```python
from build123d import *

# Parameters (mm, degrees)
SZKIC1_W                        = 203
SZKIC1_H                        = 545
DODANIE_WYCI_GNI_CIE1_DEPTH     = 1
WYTNIJ_WYCI_GNI_CIE1_DEPTH      = 437.073905415
WYTNIJ_WYCI_GNI_CIE1_DEPTH_BACK = 437.073905415
SZKIC2_W                        = 21
SZKIC2_H                        = 21
SZKIC3_W                        = 21
SZKIC3_H                        = 21
WYTNIJ_WYCI_GNI_CIE2_DEPTH      = 437.073905415
SZKIC4_W                        = 22
SZKIC4_H                        = 46.721864408
WYTNIJ_WYCI_GNI_CIE3_DEPTH      = 437.073905415
SZKIC5_W                        = 161
SZKIC5_H                        = 1
DODANIE_WYCI_GNI_CIE2_DEPTH     = 1.5
SZKIC6_R                        = 2.1
WYTNIJ_WYCI_GNI_CIE4_DEPTH      = 437.073905415
SZKIC7_R                        = 2.45
WYTNIJ_WYCI_GNI_CIE5_DEPTH      = 437.073905415
SZKIC8_W                        = 1
SZKIC8_H                        = 218.015474914
DODANIE_WYCI_GNI_CIE3_DEPTH     = 1.5
SZKIC9_W                        = 1
SZKIC9_H                        = 237.530488001
DODANIE_WYCI_GNI_CIE4_DEPTH     = 1.5
SZKIC10_R                       = 2
SZKIC10_R_2                     = 1.651116854
SZKIC10_R_3                     = 1.6
SZKIC10_R_4                     = 2.1
SZKIC10_R_5                     = 1.9
WYTNIJ_WYCI_GNI_CIE6_DEPTH      = 437.476994539
SZKIC11_R                       = 1.6
WYTNIJ_WYCI_GNI_CIE7_DEPTH      = 437.476994539
SZKIC12_R                       = 1.6
WYTNIJ_WYCI_GNI_CIE8_DEPTH      = 437.476994539


with BuildPart() as part:
    # Szkic1 → Dodanie-wyciągnięcie1 (new body)
    with BuildSketch(Plane.XY):
        with Locations((-14.988592715, -147.725961538)):
            Rectangle(SZKIC1_W, SZKIC1_H)
    extrude(amount=DODANIE_WYCI_GNI_CIE1_DEPTH)

    # Szkic2 → Wytnij-wyciągnięcie1 (cut, two sides: drawn at the far end of the back side and taken through both)
    with BuildSketch(Plane.XY.offset(1).offset(-WYTNIJ_WYCI_GNI_CIE1_DEPTH_BACK)):
        with Locations((-105.988592715, 114.274038462)):
            Rectangle(SZKIC2_W, SZKIC2_H)
        with Locations((76.011407285, 114.274038462)):
            Rectangle(SZKIC2_W, SZKIC2_H)
    extrude(amount=WYTNIJ_WYCI_GNI_CIE1_DEPTH + WYTNIJ_WYCI_GNI_CIE1_DEPTH_BACK, mode=Mode.SUBTRACT)

    # Szkic3 → Wytnij-wyciągnięcie2 (cut, through all)
    with BuildSketch(Plane.XY.offset(1)):
        with Locations((76.011407285, -409.725961538)):
            Rectangle(SZKIC3_W, SZKIC3_H)
        with Locations((-105.988592715, -409.725961538)):
            Rectangle(SZKIC3_W, SZKIC3_H)
    extrude(amount=-WYTNIJ_WYCI_GNI_CIE2_DEPTH, mode=Mode.SUBTRACT)

    # Szkic4 → Wytnij-wyciągnięcie3 (cut, through all)
    with BuildSketch(Plane.XY.offset(1)):
        with Locations((-105.488592715, -137.602368656)):
            Rectangle(SZKIC4_W, SZKIC4_H)
    extrude(amount=-WYTNIJ_WYCI_GNI_CIE3_DEPTH, mode=Mode.SUBTRACT)

    # Szkic5 → Dodanie-wyciągnięcie2 (add)
    with BuildSketch(Plane(origin=(0, 124.774038462, 0), x_dir=(1, 0, 0), z_dir=(0, 1, 0))):
        with Locations((-14.988592715, -0.5)):
            Rectangle(SZKIC5_W, SZKIC5_H)
    extrude(amount=DODANIE_WYCI_GNI_CIE2_DEPTH)

    # Szkic6 → Wytnij-wyciągnięcie4 (cut, through all)
    with BuildSketch(Plane.XY.offset(1)):
        with Locations((22.411407285, -29.125961538)):
            Circle(SZKIC6_R)
        with Locations((22.411407285, 121.674038462)):
            Circle(SZKIC6_R)
        with Locations((-88.388592715, 121.674038462)):
            Circle(SZKIC6_R)
        with Locations((-88.388592715, -29.125961538)):
            Circle(SZKIC6_R)
    extrude(amount=-WYTNIJ_WYCI_GNI_CIE4_DEPTH, mode=Mode.SUBTRACT)

    # Szkic7 → Wytnij-wyciągnięcie5 (cut, through all)
    with BuildSketch(Plane.XY.offset(1)):
        with Locations((-50.438592715, -84.464522811)):
            Circle(SZKIC7_R)
        with Locations((24.061407285, -84.464522811)):
            Circle(SZKIC7_R)
        with Locations((44.772846012, -73.225961538)):
            Circle(SZKIC7_R)
        with Locations((44.772846012, -147.725961538)):
            Circle(SZKIC7_R)
    extrude(amount=-WYTNIJ_WYCI_GNI_CIE5_DEPTH, mode=Mode.SUBTRACT)

    # Szkic8 → Dodanie-wyciągnięcie3 (add)
    with BuildSketch(Plane.ZY.offset(116.488592715)):
        with Locations((0.5, -5.233698995)):
            Rectangle(SZKIC8_W, SZKIC8_H)
    extrude(amount=DODANIE_WYCI_GNI_CIE3_DEPTH)

    # Szkic9 → Dodanie-wyciągnięcie4 (add)
    with BuildSketch(Plane.ZY.offset(116.488592715)):
        with Locations((0.5, -280.460717538)):
            Rectangle(SZKIC9_W, SZKIC9_H)
    extrude(amount=DODANIE_WYCI_GNI_CIE4_DEPTH)

    # Szkic10 → Wytnij-wyciągnięcie6 (cut, through all)
    with BuildSketch(Plane.XY.offset(1)):
        with Locations((22.211407285, -186.041328015)):
            Circle(SZKIC10_R)
        with Locations((22.662524139, -195.692444868)):
            Circle(SZKIC10_R_2)
        with Locations((-87.738592715, -186.041328015)):
            Circle(SZKIC10_R)
        with Locations((-85.588592715, -195.641328015)):
            Circle(SZKIC10_R_3)
        with Locations((-85.588592715, -380.941328015)):
            Circle(SZKIC10_R_3)
        with Locations((22.611407285, -380.941328015)):
            Circle(SZKIC10_R_3)
        with Locations((22.011407285, -416.791328015)):
            Circle(SZKIC10_R_4)
        with Locations((-87.888592715, -416.791328015)):
            Circle(SZKIC10_R_5)
    extrude(amount=-WYTNIJ_WYCI_GNI_CIE6_DEPTH, mode=Mode.SUBTRACT)

    # Szkic11 → Wytnij-wyciągnięcie7 (cut, through all)
    with BuildSketch(Plane(origin=(0, 0, 0), x_dir=(-1, 0, 0), z_dir=(0, 0, -1))):
        with Locations((4.325302662, -147.725961538)):
            Circle(SZKIC11_R)
        with Locations((69.987506483, -147.725961538)):
            Circle(SZKIC11_R)
        with Locations((-78.011407285, -147.725961538)):
            Circle(SZKIC11_R)
    extrude(amount=-WYTNIJ_WYCI_GNI_CIE7_DEPTH, mode=Mode.SUBTRACT)

    # Szkic12 → Wytnij-wyciągnięcie8 (cut, through all)
    with BuildSketch(Plane.XY.offset(1)):
        with Locations((-107.988592715, -87.725961538)):
            Circle(SZKIC12_R)
        with Locations((-107.988592715, -27.725961538)):
            Circle(SZKIC12_R)
        with Locations((-107.988592715, 32.274038462)):
            Circle(SZKIC12_R)
        with Locations((-107.988592715, 92.274038462)):
            Circle(SZKIC12_R)
        with Locations((-107.988592715, -207.725961538)):
            Circle(SZKIC12_R)
        with Locations((-107.988592715, -267.725961538)):
            Circle(SZKIC12_R)
        with Locations((-107.988592715, -327.725961538)):
            Circle(SZKIC12_R)
        with Locations((-107.988592715, -387.725961538)):
            Circle(SZKIC12_R)
        with Locations((78.011407285, 92.274038462)):
            Circle(SZKIC12_R)
        with Locations((78.011407285, 32.274038462)):
            Circle(SZKIC12_R)
        with Locations((78.011407285, -27.725961538)):
            Circle(SZKIC12_R)
        with Locations((78.011407285, -87.725961538)):
            Circle(SZKIC12_R)
        with Locations((78.011407285, -207.725961538)):
            Circle(SZKIC12_R)
        with Locations((78.011407285, -267.725961538)):
            Circle(SZKIC12_R)
        with Locations((78.011407285, -327.725961538)):
            Circle(SZKIC12_R)
        with Locations((78.011407285, -387.725961538)):
            Circle(SZKIC12_R)
        with Locations((49.40530762, 116.274038462)):
            Circle(SZKIC12_R)
        with Locations((49.40530762, -411.725961538)):
            Circle(SZKIC12_R)
    extrude(amount=-WYTNIJ_WYCI_GNI_CIE8_DEPTH, mode=Mode.SUBTRACT)


solid = part.part
```
Check sheet for the modelled part. Datum: model origin and axes. Units: mm. Round coordinates to 2 decimals unless told otherwise and drop trailing zeros. Order: outer loops, then holes, each group sorted by start corner. A loop starts at its lowest first (then second) coordinate and runs counter-clockwise, first axis right, second up.
1) Section check A-A (x = -101). Record the boundary of the cut face in (y, z).
2) Scan lines: line 1 (X direction, y = -85.5, z = 0.75); line 2 (X direction, y = -75, z = 0.95); line 3 (X direction, y = -158, z = 0.25). Record each from-to range of solid material in increasing order.
3) Section check B-B (z = 0.85). Give the number of separate pieces and of enclosed holes in the cut face, and give its area (3 significant figures).
4) Go/stop test with flat-tipped pins: pin 1 Ø4.5 at (x, y) = (24.06, -84.46) entering from -Z; pin 2 Ø0.5 at (x, z) = (-102, 0.5) entering from +Y. Record where each tip stops, or that it passes through.
Result:
1. outline: (-399.23, 0) - (-160.96, 0) - (-160.96, 1) - (-399.23, 1) - close; (-114.24, 0) - (103.77, 0) - (103.77, 1) - (-114.24, 1) - close
2. line 1: x = -117.99 to -52.66, -48.22 to 21.84, 26.28 to 86.51
2. line 2: x = -117.99 to 43.08, 46.46 to 86.51
2. line 3: x = -94.49 to 86.51
3. separate pieces: 1
3. enclosed holes: 37
3. area: 108,000 mm2
4. pin 1: passes through
4. pin 2: stops at y = 103.77
